CAD build for the part. Positions are in the model's coordinates, mm. Coordinates: 2 decimals unless noted, no trailing zeros. Order: outer loops, then holes, each group sorted by start corner. A loop starts at its lowest first (then second) coordinate and runs counter-clockwise, first axis right, second up. Notation, with made-up numbers: (-29.5, -25) - (-22.5, -25) arc R18 ccw to (-22.5, 1) - close; hole circle Ø10 at (82.5, 18). An arc over 180 degrees is marked (long way). Use one line per item in the form item = value.
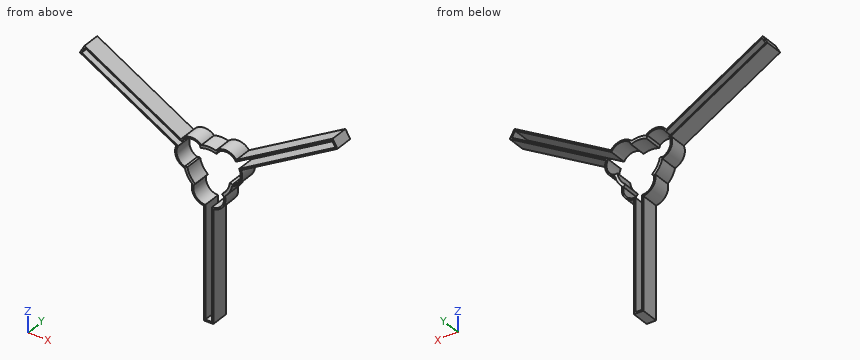
```python
from build123d import *

# Parameters (mm, degrees)
BOSS_EXTRUDE1_DEPTH = 15


with BuildPart() as part:
    # Sketch1 → Boss-Extrude1 (new body)
    with BuildSketch(Plane(origin=(0, 0, 0), x_dir=(1, 0, 0), z_dir=(0, 1, 0))):
        with BuildLine():
            ThreePointArc((12.518734156, 15.597477204), (13.041444472, 15.163137079), (13.549095916, 14.711288178))
            ThreePointArc((13.549095916, 14.711288178), (11.904160472, 23.874346891), (3.9, 28.62838441))
            Line((3.9, 28.62838441), (3.9, 120.5))
            Line((3.9, 120.5), (0, 120.5))
            Line((0, 120.5), (-3.9, 120.5))
            Line((-3.9, 120.5), (-3.9, 28.62838441))
            ThreePointArc((-3.9, 28.62838441), (-11.904160472, 23.874346891), (-13.549095916, 14.711288178))
            ThreePointArc((-13.549095916, 14.711288178), (-13.041444472, 15.163137079), (-12.518734156, 15.597477204))
            ThreePointArc((-12.518734156, 15.597477204), (-10.412126322, 23.858631961), (-2.7, 27.492855685))
            Line((-2.7, 27.492855685), (-2.7, 119.3))
            Line((-2.7, 119.3), (2.7, 119.3))
            Line((2.7, 119.3), (2.7, 27.492855685))
            ThreePointArc((2.7, 27.492855685), (10.412126322, 23.858631961), (12.518734156, 15.597477204))
        make_face()
        with BuildLine():
            ThreePointArc((-17.493953036, 2.692880832), (-15.328649647, 8.85), (-11.079079728, 13.803767326))
            Line((-11.079079728, 13.803767326), (-12.518734156, 15.597477204))
            ThreePointArc((-12.518734156, 15.597477204), (-13.041444472, 15.163137079), (-13.549095916, 14.711288178))
            ThreePointArc((-13.549095916, 14.711288178), (-17.320508076, 10), (-19.514897242, 4.378217173))
            ThreePointArc((-19.514897242, 4.378217173), (-19.652384148, 3.712653675), (-19.767178572, 3.0428032))
            Line((-19.767178572, 3.0428032), (-17.493953036, 2.692880832))
        make_face()
        with BuildLine():
            ThreePointArc((-22.842908169, -17.69169128), (-14.72371067, -22.246478824), (-5.965801326, -19.089505351))
            ThreePointArc((-5.965801326, -19.089505351), (-6.610939676, -18.875790754), (-7.248444416, -18.640280404))
            ThreePointArc((-7.248444416, -18.640280404), (-15.456118217, -20.946481882), (-22.459511445, -16.084696432))
            Line((-22.459511445, -16.084696432), (-101.966830671, -61.98826859))
            Line((-101.966830671, -61.98826859), (-104.666830671, -57.31173141))
            Line((-104.666830671, -57.31173141), (-25.159511445, -11.408159252))
            ThreePointArc((-25.159511445, -11.408159252), (-25.868244538, -2.912150078), (-19.767178572, 3.0428032))
            ThreePointArc((-19.767178572, 3.0428032), (-19.652384148, 3.712653675), (-19.514897242, 4.378217173))
            ThreePointArc((-19.514897242, 4.378217173), (-26.627871142, -1.627868066), (-26.742908169, -10.93669313))
            Line((-26.742908169, -10.93669313), (-106.306061156, -56.872500925))
            Line((-106.306061156, -56.872500925), (-104.356061156, -60.25))
            Line((-104.356061156, -60.25), (-102.406061156, -63.627499075))
            Line((-102.406061156, -63.627499075), (-22.842908169, -17.69169128))
        make_face()
        with BuildLine():
            Line((17.493953036, 2.692880832), (19.767178572, 3.0428032))
            ThreePointArc((19.767178572, 3.0428032), (19.652384148, 3.712653675), (19.514897242, 4.378217173))
            ThreePointArc((19.514897242, 4.378217173), (17.320508076, 10), (13.549095916, 14.711288178))
            ThreePointArc((13.549095916, 14.711288178), (13.041444472, 15.163137079), (12.518734156, 15.597477204))
            Line((12.518734156, 15.597477204), (11.079079728, 13.803767326))
            ThreePointArc((11.079079728, 13.803767326), (15.328649647, 8.85), (17.493953036, 2.692880832))
        make_face()
        with BuildLine():
            ThreePointArc((5.965801326, -19.089505351), (6.610939676, -18.875790754), (7.248444416, -18.640280404))
            Line((7.248444416, -18.640280404), (6.414873308, -16.496648158))
            ThreePointArc((6.414873308, -16.496648158), (0, -17.7), (-6.414873308, -16.496648158))
            Line((-6.414873308, -16.496648158), (-7.248444416, -18.640280404))
            ThreePointArc((-7.248444416, -18.640280404), (-6.610939676, -18.875790754), (-5.965801326, -19.089505351))
            ThreePointArc((-5.965801326, -19.089505351), (0, -20), (5.965801326, -19.089505351))
        make_face()
        with BuildLine():
            ThreePointArc((19.767178572, 3.0428032), (25.868244538, -2.912150078), (25.159511445, -11.408159252))
            Line((25.159511445, -11.408159252), (104.666830671, -57.31173141))
            Line((104.666830671, -57.31173141), (101.966830671, -61.98826859))
            Line((101.966830671, -61.98826859), (22.459511445, -16.084696432))
            ThreePointArc((22.459511445, -16.084696432), (15.456118217, -20.946481882), (7.248444416, -18.640280404))
            ThreePointArc((7.248444416, -18.640280404), (6.610939676, -18.875790754), (5.965801326, -19.089505351))
            ThreePointArc((5.965801326, -19.089505351), (14.72371067, -22.246478824), (22.842908169, -17.69169128))
            Line((22.842908169, -17.69169128), (102.406061156, -63.627499075))
            Line((102.406061156, -63.627499075), (104.356061156, -60.25))
            Line((104.356061156, -60.25), (106.306061156, -56.872500925))
            Line((106.306061156, -56.872500925), (26.742908169, -10.93669313))
            ThreePointArc((26.742908169, -10.93669313), (26.627871142, -1.627868066), (19.514897242, 4.378217173))
            ThreePointArc((19.514897242, 4.378217173), (19.652384148, 3.712653675), (19.767178572, 3.0428032))
        make_face()
    extrude(amount=BOSS_EXTRUDE1_DEPTH)


solid = part.part
```
Item 1: Drop flat-ended pins along their axis: pin 1 (1.6 mm diameter, centred on x = 1, y = 10, fed in from +Z); pin 2 (2 mm diameter, centred on x = 59.5, y = 12.5, fed in from +Z); pin 3 (2 mm diameter, centred on x = 62, y = 3, fed in from -Z). Give the stop position or say it passes through.
Derived:
pin_1 = 20
pin_2 = 39.43
pin_3 = 30.72
Item 2: Drill centre lines: line 1 (X direction, y = 12.5, z = -36); line 2 (X direction, y = 10.75, z = 55.5); line 3 (X direction, y = 6.75, z = 27). Where is each one in solid material? Low to high. Write a range as [from, to].
Derived:
line_1 = [-3.9, -2.7], [2.7, 3.9]
line_2 = [-103.93, -101.53], [-90.73, -88.33], [88.33, 90.73], [101.53, 103.93]
line_3 = [-54.57, -52.17], [-41.37, -38.97], [38.97, 41.37], [52.17, 54.57]
Item 3: Cut at B-B, the plane z = 37.5. Write the cut outline in (x, y).
Derived:
outline = (-72.75, 0) - (-70.35, 0) - (-70.35, 15) - (-72.75, 15) - close; (-59.55, 0) - (-57.15, 0) - (-57.15, 15) - (-59.55, 15) - close; (57.15, 0) - (59.55, 0) - (59.55, 15) - (57.15, 15) - close; (70.35, 0) - (72.75, 0) - (72.75, 15) - (70.35, 15) - close
Item 4: Cut at A-A, the plane z = -76. Write the cut outline in (x, y).
Derived:
outline = (-3.9, 0) - (-2.7, 0) - (-2.7, 15) - (-3.9, 15) - close; (2.7, 0) - (3.9, 0) - (3.9, 15) - (2.7, 15) - close
Item 5: Cut at C-C, the plane x = -86. Write the cut outline in (y, z).
Derived:
outline = (0, 45.15) - (15, 45.15) - (15, 46.53) - (0, 46.53) - close; (0, 52.77) - (15, 52.77) - (15, 54.16) - (0, 54.16) - close
